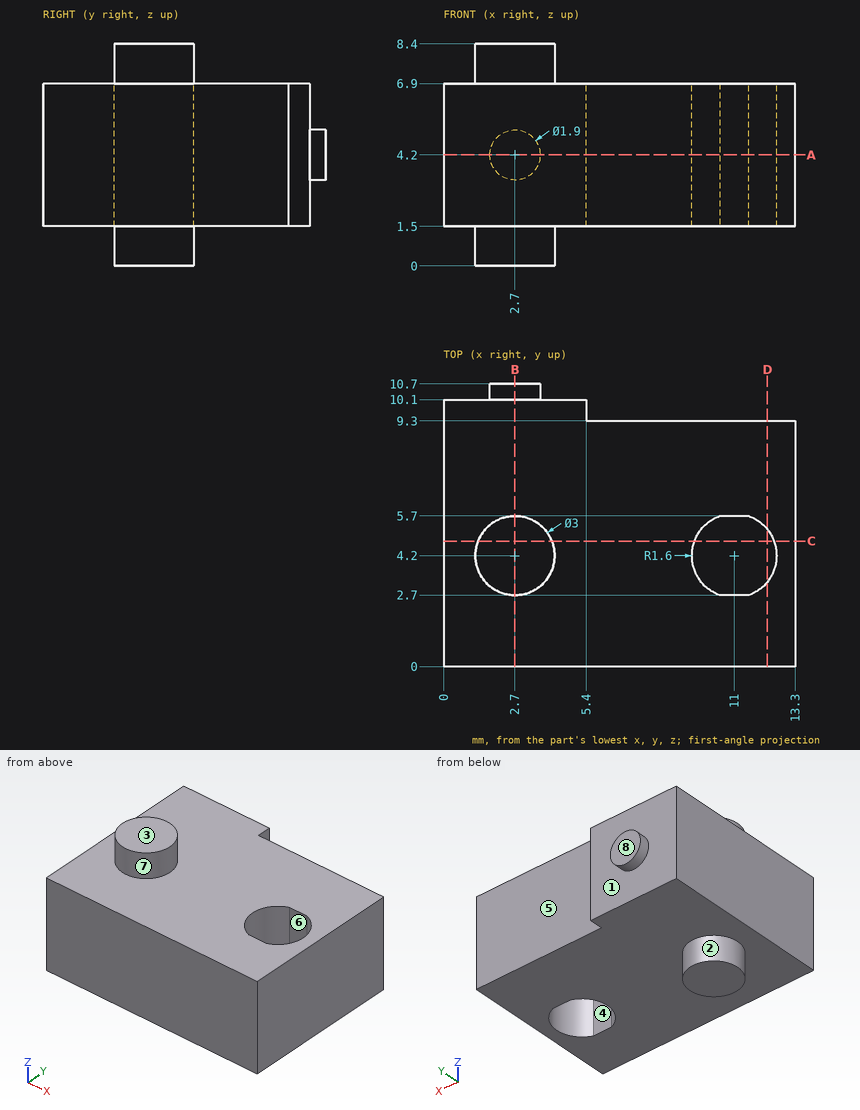
Answer from the drawing. Dimensions are ordinates in mm from the lowest x, y and z of the part. A direction names the side the tool comes from. Give positions to 0.01 mm unless a question says otherwise; leave off trailing zeros. Order: outer loops, then holes, each group sorted by start corner. A loop starts at its lowest first (then second) coordinate and runs counter-clockwise, first axis right, second up.
Item 1: The part is cut by section D-D, the plane x = 12.25. Give the vertices of the cut face in (y, z).
From the geometry:
outline: (0, 1.5) - (3.2, 1.5) - (3.2, 6.9) - (0, 6.9) - close; (5.2, 1.5) - (9.3, 1.5) - (9.3, 6.9) - (5.2, 6.9) - close
Item 2: Find the intervals of material crossed by probe 1 along Y at (x, z) = (11.25, 2.5); probe 2 along Z at (x, y) = (12, 1.75); probe 3 along Y at (x, z) = (7.25, 6.5), in increasing order.
From the geometry:
probe 1: y = 0 to 2.7, 5.7 to 9.3
probe 2: z = 1.5 to 6.9
probe 3: y = 0 to 9.3
Item 3: Given pin 1 Ø0.6 at (y, z) = (9.5, 5) entering from +X; pin 2 Ø3 at (x, y) = (9, 6) entering from +Z; pin 3 Ø2.5 at (x, z) = (11, 4) entering from +Y; pin 4 Ø5 at (x, y) = (7.5, 3) entering from -Z, each flat-ended and moving along its own axis, determine where each tip first touches the part or whether it passes through.
From the geometry:
pin 1: stops at x = 13.3
pin 2: stops at z = 6.9
pin 3: stops at y = 9.3
pin 4: stops at z = 1.5
Item 4: Which of the six approach directions +Z, -Z, +X, -X, +Y, -Y give full straight-line access (tool end or side, diameter ignored) to the marked faces 1, 2, 3, 4 and 5?
From the geometry:
face 1: +Y
face 2: -Z
face 3: +Z, +X, -X, +Y, -Y
face 4: +Z, -Z
face 5: +Z, -Z, +X, +Y
Item 5: The part is cut by section C-C, the plane y = 4.75. Give the vertices of the cut face in (x, z).
From the geometry:
outline: (0, 1.5) - (1.3, 1.5) - (1.3, 0) - (4.1, 0) - (4.1, 1.5) - (9.5, 1.5) - (9.5, 6.9) - (4.1, 6.9) - (4.1, 8.4) - (1.3, 8.4) - (1.3, 6.9) - (0, 6.9) - close; (12.5, 1.5) - (13.3, 1.5) - (13.3, 6.9) - (12.5, 6.9) - close
Item 6: The part is cut by section A-A, the plane z = 4.2. Give the vertices of the cut face in (x, y).
From the geometry:
outline: (0, 0) - (13.3, 0) - (13.3, 9.3) - (5.4, 9.3) - (5.4, 10.1) - (3.65, 10.1) - (3.65, 10.7) - (1.75, 10.7) - (1.75, 10.1) - (0, 10.1) - close; hole (10.44, 2.7) - (11.56, 2.7) arc R1.6 ccw to (11.56, 5.7) - (10.44, 5.7) arc R1.6 ccw to start
Item 7: For a pull along X with two mould halves and no side action, classify the marked faces 6, 7 and 8 as pulls with the +X half, pulls with the -X half, needs draft (parallel to the pull), parting line crosses it, or undercut.
From the geometry:
face 6: undercut
face 7: parting line crosses it
face 8: needs draft
Item 8: The part is cut by section B-B, the plane x = 2.7. Give the vertices of the cut face in (y, z).
From the geometry:
outline: (0, 1.5) - (2.7, 1.5) - (2.7, 0) - (5.7, 0) - (5.7, 1.5) - (10.1, 1.5) - (10.1, 3.25) - (10.7, 3.25) - (10.7, 5.15) - (10.1, 5.15) - (10.1, 6.9) - (5.7, 6.9) - (5.7, 8.4) - (2.7, 8.4) - (2.7, 6.9) - (0, 6.9) - close
